Autodesk Fusion 360 part; units mm, degrees
sketch "Sketch1" plane through (0, 0, 0) normal (0, 1, 0) x (1, 0, 0)
  line L0 (25, -92) -> (83, -92)
  line L1 (83, -92) -> (83, 0)
  line L2 (83, 0) -> (25, 0)
  line L3 (54, -92) -> (25, -92)
  line L4 (54, -92) -> (83, -92)
  line L5 (-6, -92) -> (-6, 24)
  line L6 (-6, 24) -> (114, 24)
  line L7 (114, 24) -> (114, -106)
  line L8 (104, -116) -> (4, -116)
  line L9 (-6, -106) -> (-6, -92)
  line L10 (25, -92) -> (25, 0)
  arc A0 (104, -116) -> (114, -106) centre (104, -106) ccw
  arc A1 (-6, -106) -> (4, -116) centre (4, -106) ccw
  line L11 (110, -110) -> (110, 20)
  line L12 (-6, 11.8684) -> (-2, 11.8684)
  line L13 (110, 20) -> (-2, 20)
  line L14 (-2, 20) -> (-2, -110)
  line L15 (-2, -110) -> (110, -110)
  dimension "d1" = 92
  dimension "d3" = 60
  dimension "d7" = 10
  dimension "d8" = 10
sketch "Sketch2" plane through (0, 0, 0) normal (0, 1, 0) x (1, 0, 0)
  line L0 (114, 24) -> (114, 64)
  line L1 (114, 64) -> (-6, 64)
  line L2 (-6, 64) -> (-6, 24)
  line L3 (-2, 24) -> (-2, 60)
  line L4 (-2, 60) -> (110, 60)
  line L5 (110, 60) -> (110, 24)
  line L6 (114, 24) -> (110, 24)
  line L7 (-2, 24) -> (-6, 24)
  line L8 (114, 64) -> (114, 94)
  line L9 (114, 94) -> (-6, 94)
  line L10 (-6, 94) -> (-6, 64)
  line L11 (-2, 64) -> (-2, 90)
  line L12 (110, 64) -> (110, 90)
  line L13 (110, 90) -> (-2, 90)
  line L14 (110, 90) -> (114, 90)
  line L15 (-2, 90) -> (-6, 90)
  dimension "d13" = 40
  dimension "d18" = 30
  dimension "d19" = 26
  dimension "d20" = 26
sketch "Sketch3" plane through (0, 0, -20) normal (0, 0, 1) x (-1, 0, 0)
  line L0 (-110, 0) -> (2, 0)
  line L1 (2, 0) -> (2, 90)
  line L2 (2, 90) -> (-110, 90)
  line L3 (-110, 90) -> (-110, 0)
  line L4 (-35, 65) -> (-80, 65)
  line L5 (-80, 65) -> (-80, 75)
  line L6 (-80, 75) -> (-35, 75)
  line L7 (-35, 75) -> (-35, 65)
sketch "Sketch4" plane through (0, 1.5, 0) normal (0, 1, 0) x (-1, 0, 0)
  line L0 (-83, 92) -> (-25, 92)
  line L1 (-25, 92) -> (-25, 0)
  line L2 (-25, 0) -> (-83, 0)
  line L3 (-83, 0) -> (-83, 92)
  line L4 (2, 110) -> (-110, 110)
  line L5 (-110, 110) -> (-110, -20)
  line L6 (-110, -20) -> (2, -20)
  line L7 (2, -20) -> (2, 110)
extrude "Extrude6" add sketch "Sketch1" against normal blind 1.5 contours L11 L13 L14 L15
extrude "Extrude7" add sketch "Sketch1" sketch "Sketch2" against normal blind 90 contours L5 L6 L7 L8 L9 A0 A1 of sketch 2 contours L0 L1 L2 L3 L4 L5 L6 L7 | L1 L8 L12 L14 | L8 L9 L10 L13 L14 L15 | L1 L10 L11 L15
extrude "Extrude8" add sketch "Sketch2" along normal blind 30 contours L8 L9 L10 L13 L14 L15
sketch "Sketch5" plane through (0, 0, -20) normal (0, 0, 1) x (-1, 0, 0)
  line L0 (-110, 1.5) -> (2, 1.5)
  line L1 (2, 1.5) -> (2, 90)
  line L2 (2, 90) -> (-110, 90)
  line L3 (-110, 90) -> (-110, 1.5)
  line L4 (-5, 20) -> (-5, 65)
  line L5 (-5, 65) -> (-10, 65)
  line L6 (-10, 65) -> (-10, 20)
  line L7 (-10, 20) -> (-5, 20)
  line L8 (-105, 20) -> (-105, 65)
  line L9 (-105, 65) -> (-100, 65)
  line L10 (-100, 65) -> (-100, 20)
  line L11 (-100, 20) -> (-105, 20)
extrude "Extrude9" cut sketch "Sketch5" against normal blind 44 contours L4 L5 L6 L7 | L8 L9 L10 L11
sketch "Sketch6" plane through (0, 1.5, 0) normal (0, 1, 0) x (-1, 0, 0)
  circle A0 centre (-91.2, 46.0087) radius 1.5
  circle A1 centre (-14.7, 45.9255) radius 1.5
  dimension "d32" = 3
  dimension "d35" = 3
extrude "Extrude10" add sketch "Sketch4" against normal blind 3
extrude "Extrude11" cut sketch "Sketch6" against normal blind 3
extrude "Extrude12" cut 1 faces at (12.2549, 1.5, 83.0328) along direction (0, -1, 0) blind 3
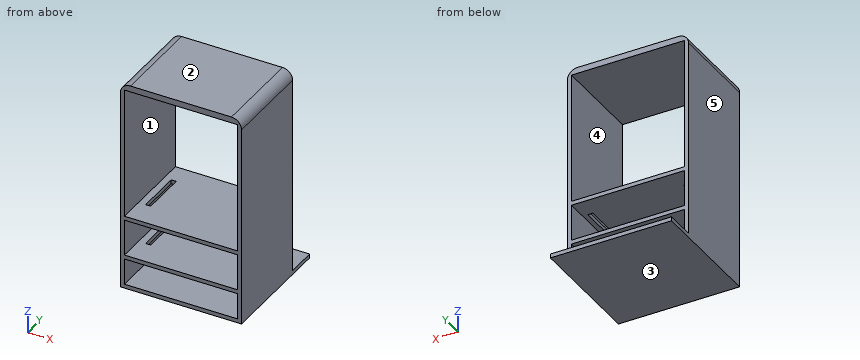
CAD build for the part. Positions are in the model's coordinates, mm. Face numbers are marked on the shaded views. A direction names the side the tool comes from. Give positions to 0.01 mm unless a question says otherwise; leave off trailing zeros. Write each loop counter-clockwise with the first axis right and the second up, starting at its lowest first coordinate (ties: lowest second). Pieces come first, ordered by that corner, then holes. Notation, with made-up numbers: M -27,47.5 L -12,47.5 A23 cw -12,68.5 Z; hole C 5.5,-7.5 d4. An arc over 180 degrees is marked long. Return JSON: item names as keys, results as strings. Group by question number.
(1) Band-saw the part on D-D (y = -72). Give the cut face in (x, z), and give its area (3 significant figures).
(2) Drill centre lines: L1, parallel to Z at x = 91.5, y = -41; L2, parallel to X at y = -74, z = 21.5; L3, parallel to Z at x = 16.5, y = 21. Where is each one in solid material? Low to high. Write a range as [from, to].
(3) Band-saw the part on A-A (y = -58). State how many separate pieces and enclosed holes the cut face has, and give its area (3 significant figures).
(4) Band-saw the part on B-B (x = 35). Give the cut face in (y, z).
(5) Flat gauge pin, fed straight in: pin 1 Ø2 at (x, z) = (8.5, -22) entering from +Y. Where does the tip first touch, or does it go through?
(6) Mould opens along X. For the marked faces 3, 4 and 5 say: pulls with the +X half, pulls with the -X half, needs draft (parallel to the pull), parting line crosses it, or undercut.
(7) Band-saw the part on C-C (z = -55.5). Give the cut face in (x, y).
(8) 3-axis set-ups, long thin cutter, end or side, ignore diameter. For the marked faces 1 and 2: which of +Z, -Z, +X, -X, +Y, -Y reach the whole face in a straight line?
Entries:
{
 "1": {"outline": "M -6,-94 L 114,-94 L 114,106 A10 ccw 104,116 L 4,116 A10 ccw -6,106 Z; hole M -2,-90 L 110,-90 L 110,-64 L -2,-64 Z; hole M -2,-60 L 110,-60 L 110,-24 L -2,-24 Z; hole M -2,-20 L 110,-20 L 110,110 L -2,110 Z", "area": "3,650 mm^2"},
 "2": {"L1": "z = [-94, -90], [-64, -60], [-24, -20], [110, 116]", "L2": "x = [-6, -2], [110, 114]", "L3": "z = [-94, -90]"},
 "3": {"separate pieces": "3", "enclosed holes": "1", "area": "3,570 mm^2"},
 "4": {"outline": "M -90,-94 L 30,-94 L 30,-90 L -90,-90 Z; M -90,-64 L 0,-64 L 0,-60 L -90,-60 Z; M -90,-24 L 0,-24 L 0,-20 L -90,-20 Z; M -90,110 L 0,110 L 0,116 L -90,116 Z"},
 "5": {"pin 1": "stops at y = 0"},
 "6": {"face 3": "needs draft", "face 4": "undercut", "face 5": "pulls with the -X half"},
 "7": {"outline": "M -6,-90 L -2,-90 L -2,0 L -6,0 Z; M 110,-90 L 114,-90 L 114,0 L 110,0 Z"},
 "8": {"face 1": "+Y, -Y", "face 2": "+Z, +X, -X, +Y, -Y"}
}
